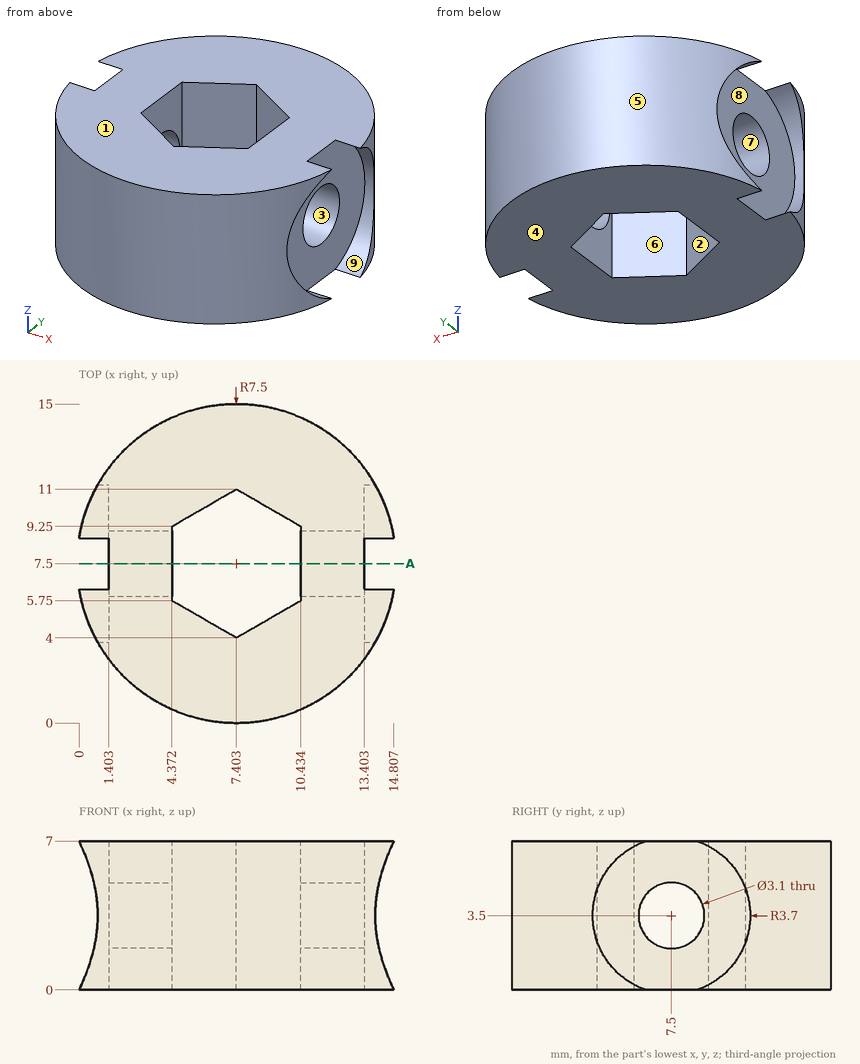
Answer from the drawing. Dimensions are ordinates in mm from the lowest x, y and z of the part. A direction names the side the tool comes from. Round coordinates to 2 decimals unless told otherwise and drop trailing zeros.
1) For the marked faces 5, 6, 7, 8 and 9, determine the directions among +Z, -Z, +X, -X, +Y, -Y from which every point of the face is accessible in a straight line to the end or side of a thin tool.
2) The part is cut by section A-A on y = 7.5. Give the number of separate pieces and of enclosed holes in the cut face.
3) Flat-ended cylindrical pins translate along their axes: pin 1 (1.1 mm diameter, centred on y = 8, z = 2.5, fed in from +X); pin 2 (4 mm diameter, centred on y = 7.5, z = 4, fed in from -X); pin 3 (1 mm diameter, centred on y = 7.5, z = 3, fed in from -X); pin 4 (4 mm diameter, centred on x = 4, z = 5.5, fed in from -Y). Find the tip coordinate at first contact, or state that the pin passes through.
4) Straight lines are drawn through the part: L1, parallel to X at y = 9, z = 1.5 (1 decimal); L2, parallel to Y at x = 14, z = 1 (1 decimal); L3, parallel to Y at x = 5.25, z = 1.75 (1 decimal). For each, find the intervals that lie inside material, in ascending order.
5) The mould has two halves that part along Z. Classify the marked faces 1, 2, 3 and 4: released by +Z, released by -Z, zero draft, split by the parting line, or undercut.
Resolved:
1. face 5: +Z, -Z, +Y
1. face 6: +Z, -Z
1. face 7: +X, -X
1. face 8: -X
1. face 9: +X
2. separate pieces: 4
2. enclosed holes: 0
3. pin 1: stops at x = 13.4
3. pin 2: stops at x = 1.4
3. pin 3: passes through
3. pin 4: stops at y = 0.13
4. L1: x = 1.4 to 4.4, 10.4 to 13.4
4. L2: y = 3.9 to 4.8, 10.2 to 11.1
4. L3: y = 0.3 to 5.2, 9.8 to 14.7
5. face 1: released by +Z
5. face 2: zero draft
5. face 3: undercut
5. face 4: released by -Z
